from build123d import *

# Parameters (mm, degrees)
SKETCH_1_R      = 1.55
EXTRUDE_1_DEPTH = 3


with BuildPart() as part:
    # 草图1 → 凸台-拉伸1 (new body)
    with BuildSketch(Plane(origin=(0, 0, 0), x_dir=(0, 0, -1), z_dir=(1, 0, 0))):
        with BuildLine():
            Line((-2.008575125, 4), (4.438262309, 4))
            ThreePointArc((4.438262309, 4), (7.612856223, 4.710298), (10.5, 3.211308145))
            Line((10.5, 3.211308145), (10.5, -3.211308145))
            ThreePointArc((10.5, -3.211308145), (7.612856223, -4.710298), (4.438262309, -4))
            Line((4.438262309, -4), (-2.008575125, -4))
            ThreePointArc((-2.008575125, -4), (-2.671034277, -3.186336048), (-3.695652174, -3.412299143))
            ThreePointArc((-3.695652174, -3.412299143), (-7.140247241, -4.747929097), (-10.5, -3.211308145))
            Line((-10.5, -3.211308145), (-10.5, 3.211308145))
            ThreePointArc((-10.5, 3.211308145), (-7.140247241, 4.747929097), (-3.695652174, 3.412299143))
            ThreePointArc((-3.695652174, 3.412299143), (-2.671034277, 3.186336048), (-2.008575125, 4))
        make_face()
        with Locations((-7, 0)):
            Circle(SKETCH_1_R, mode=Mode.SUBTRACT)
        with Locations(Location((7, 0, 0), (0, 0, 180))):
            Circle(SKETCH_1_R, mode=Mode.SUBTRACT)
    extrude(amount=EXTRUDE_1_DEPTH)


solid = part.part
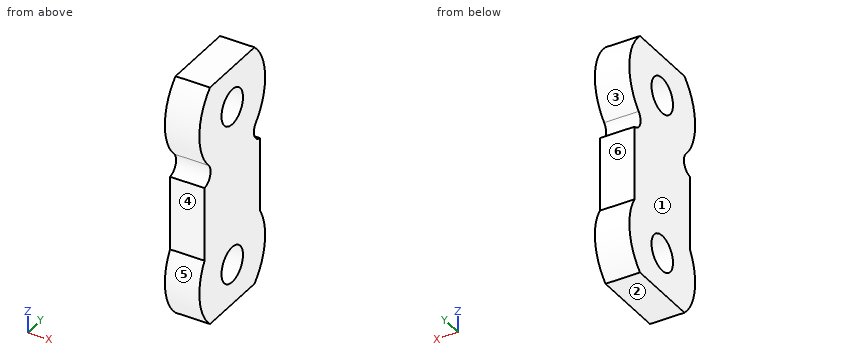
Geometry: final body of the model. Coordinates: model frame, mm. Face numbers are marked on the shaded views. A direction names the side the tool comes from. Give positions to 0.01 mm unless a question says otherwise; leave off trailing zeros. Write each loop counter-clockwise with the first axis right and the second up, starting at its lowest first coordinate (ties: lowest second). Pieces come first, ordered by that corner, then holes. Notation, with made-up numbers: (77, 10.5) -> (98, 10.5) arc R26 ccw to (98, 34.5) -> close; hole circle Ø2 at (21, 67). An arc over 180 degrees is marked (long way). Answer in a Markdown table with one row per item.
(1) Section query B-B on y = 0. Return loops of the section in (x, z).
Answers below:
| item | result |
|---|---|
| outline | (0, -10.5) -> (3, -10.5) -> (3, -8.55) -> (0, -8.55) -> close; (0, -5.45) -> (3, -5.45) -> (3, 5.45) -> (0, 5.45) -> close; (0, 8.55) -> (3, 8.55) -> (3, 10.5) -> (0, 10.5) -> close |
(2) Pin query (flat end, axial travel): pin 1 (1.9 mm diameter, centred on y = 0, z = -7, fed in from -X); pin 2 (1.5 mm diameter, centred on x = 2, z = -1.5, fed in from -Y). Return the tip coordinate at first contact, or that it passes through.
Answers below:
| item | result |
|---|---|
| pin 1 | through |
| pin 2 | y = -4 |
(3) Section query C-C on x = 0.45. Return loops of the section in (y, z), then the cut area to 3 significant figures.
Answers below:
| item | result |
|---|---|
| outline | (-4, -4.44) arc R4.75 ccw to (-3.21, -10.5) -> (3.21, -10.5) arc R4.75 ccw to (4, -4.44) -> (4, 2.01) arc R1 cw to (3.41, 3.7) arc R4.75 ccw to (3.21, 10.5) -> (-3.21, 10.5) arc R4.75 ccw to (-3.41, 3.7) arc R1 cw to (-4, 2.01) -> close; hole circle Ø3.1 at (0, -7); hole circle Ø3.1 at (0, 7) |
| area | 159 mm^2 |
(4) Draft query along Z for the marked faces 1, 2, 3 and 4. Return one class per face: +Z half, -Z half, draft (parallel to the pull), parting line (faces both ways), or undercut.
Answers below:
| item | result |
|---|---|
| face 1 | draft |
| face 2 | -Z half |
| face 3 | undercut |
| face 4 | undercut |
(5) Ray query, line 1 along Y through (x, z) = (2.25, -7); line 2 along Z through (x, y) = (1.05, -1); line 3 along Z through (x, y) = (1, 0.5). Return the intervals inside material, ascending. Write a range as [from, to].
Answers below:
| item | result |
|---|---|
| line 1 | [-4.75, -1.55], [1.55, 4.75] |
| line 2 | [-10.5, -8.18], [-5.82, 5.82], [8.18, 10.5] |
| line 3 | [-10.5, -8.47], [-5.53, 5.53], [8.47, 10.5] |
(6) Section query A-A on z = -7. Return loops of the section in (x, y), then the cut area to 3 significant figures.
Answers below:
| item | result |
|---|---|
| outline | (0, -4.75) -> (3, -4.75) -> (3, -1.55) -> (0, -1.55) -> close; (0, 1.55) -> (3, 1.55) -> (3, 4.75) -> (0, 4.75) -> close |
| area | 19.2 mm^2 |
(7) Section query D-D on z = 6.5. Return loops of the section in (x, y), then the cut area to 3 significant figures.
Answers below:
| item | result |
|---|---|
| outline | (0, -4.72) -> (3, -4.72) -> (3, -1.47) -> (0, -1.47) -> close; (0, 1.47) -> (3, 1.47) -> (3, 4.72) -> (0, 4.72) -> close |
| area | 19.5 mm^2 |
(8) Set-up query: the marked faces 5 and 6. Return all of +Z, -Z, +X, -X, +Y, -Y with unobstructed straight access to the full face (end or side cutting, diameter ignored); none if empty.
Answers below:
| item | result |
|---|---|
| face 5 | +X, -X, -Y |
| face 6 | +X, -X, +Y |
